from build123d import *

# Parameters (mm, degrees)
F0_R     = 9.85
F0_R_2   = 0.5
F0_R_3   = 1
F1_DEPTH = 1.5
F2_R     = 3
F2_R_2   = 1.8
F3_DEPTH = 2.5
F4_R     = 1.8
F4_R_2   = 1
F5_DEPTH = 0.5


with BuildPart() as f1:
    # F0 (on Top) → F1 (new body)
    with BuildSketch(Plane.XY):
        Circle(F0_R)
        with Locations((0, -8.5)):
            Circle(F0_R_2, mode=Mode.SUBTRACT)
        with Locations((0, -6.5)):
            Circle(F0_R_2, mode=Mode.SUBTRACT)
        with Locations((0, -4.5)):
            Circle(F0_R_2, mode=Mode.SUBTRACT)
        with Locations((-8.5, 0)):
            Circle(F0_R_2, mode=Mode.SUBTRACT)
        with Locations((-6.5, 0)):
            Circle(F0_R_2, mode=Mode.SUBTRACT)
        with Locations((-4.5, 0)):
            Circle(F0_R_2, mode=Mode.SUBTRACT)
        Circle(F0_R_3, mode=Mode.SUBTRACT)
        with Locations((4.5, 0)):
            Circle(F0_R_2, mode=Mode.SUBTRACT)
        with Locations((0, 4.5)):
            Circle(F0_R_2, mode=Mode.SUBTRACT)
        with Locations((6.5, 0)):
            Circle(F0_R_2, mode=Mode.SUBTRACT)
        with Locations((8.5, 0)):
            Circle(F0_R_2, mode=Mode.SUBTRACT)
        with Locations((0, 6.5)):
            Circle(F0_R_2, mode=Mode.SUBTRACT)
        with Locations((0, 8.5)):
            Circle(F0_R_2, mode=Mode.SUBTRACT)
    extrude(amount=F1_DEPTH)

    # F2 (on face) → F3 (join)
    with BuildSketch(Plane.XY.offset(1.5)):
        Circle(F2_R)
        Circle(F2_R_2, mode=Mode.SUBTRACT)
    extrude(amount=F3_DEPTH)

    # F4 (on face) → F5 (join)
    with BuildSketch(Plane.XY.offset(1.5)):
        Circle(F4_R)
        Circle(F4_R_2, mode=Mode.SUBTRACT)
    extrude(amount=F5_DEPTH)


solid = f1.part
Could you check a few things on this model? Use its own coordinates, in mm. A direction names the side the tool comes from. Give positions to 0.01 mm unless a question says otherwise; leave off trailing zeros. Write each loop counter-clockwise with the first axis right and the second up, starting at its lowest first coordinate (ties: lowest second). Pieces come first, ordered by that corner, then holes. Notation, with made-up numbers: (87.5, 31) -> (94.5, 31) arc R24 cw to (94.5, 46) -> close; hole circle Ø6 at (43, -28). An arc over 180 degrees is marked (long way). Answer as a JSON object with one key per item and string values.
Q1. Which directions (+Z, -Z, +X, -X, +Y, -Y) give clear straight access to the entire face, cutting with the end or side of a thin tool? Please do faces 1 (the flat face through (-2.3, 2.3, 1.5)), 2 (the cylindrical face through (0, -4, 1)).
Taken from the geometry:
{"face 1": "+Z", "face 2": "+Z, -Z"}
Q2. We'd pull the mould along Y, two halves only. Please class faces 3 (the flat face through (0, -2, 4)), 4 (the cylindrical face through (-7.82, -5.99, 0.74)), 5 (the cylindrical face through (-5, 0, 1)): released by +Y, released by -Y, zero draft, split by the parting line, or undercut.
Taken from the geometry:
{"face 3": "zero draft", "face 4": "split by the parting line", "face 5": "undercut"}
Q3. Will these pins go through, and if not, where does the flat tip stop? pin 1 Ø3 at (x, y) = (0, 0.5) entering from +Z; pin 2 Ø1.5 at (x, z) = (2, 0.5) entering from -Y; pin 3 Ø2 at (x, z) = (0, 3.5) entering from +Y; pin 4 Ø3 at (x, y) = (0, 0) entering from +Z.
Taken from the geometry:
{"pin 1": "stops at z = 4", "pin 2": "stops at y = -9.77", "pin 3": "stops at y = 3", "pin 4": "stops at z = 2"}
Q4. Suppose I cut it at C-C on y = 0. Count the separate pieces of the cut face and the enclosed holes in it, then the cut area to 4 significant figures.
Taken from the geometry:
{"separate pieces": "8", "enclosed holes": "0", "area": "24.35 mm²"}
Q5. Suppose I cut it at D-D on z = 2.8. Write out the boundary of the cut face in (x, y).
Taken from the geometry:
{"outline": "circle Ø6 at (0, 0); hole circle Ø3.6 at (0, 0)"}
Q6. Suppose I cut it at A-A on x = 8.25. Write out the boundary of the cut face in (y, z), then the cut area to 3 significant figures.
Taken from the geometry:
{"outline": "(-5.38, 0) -> (-0.43, 0) -> (-0.43, 1.5) -> (-5.38, 1.5) -> close; (0.43, 0) -> (5.38, 0) -> (5.38, 1.5) -> (0.43, 1.5) -> close", "area": "14.8 mm²"}
Q7. Please list where these lines run through material, in increasing order: L1, parallel to Z at x = 0.5, y = -1; L2, parallel to Z at x = -7.5, y = 6; L3, parallel to Y at x = 0.75, z = 1.8.
Taken from the geometry:
{"L1": "z = 0 to 2", "L2": "z = 0 to 1.5", "L3": "y = -2.9 to -0.66, 0.66 to 2.9"}
Q8. Suppose I cut it at B-B on y = 4.5. Write out the boundary of the cut face in (x, z), then the cut area to 3 significant figures.
Taken from the geometry:
{"outline": "(-8.76, 0) -> (-0.5, 0) -> (-0.5, 1.5) -> (-8.76, 1.5) -> close; (0.5, 0) -> (8.76, 0) -> (8.76, 1.5) -> (0.5, 1.5) -> close", "area": "24.8 mm²"}
